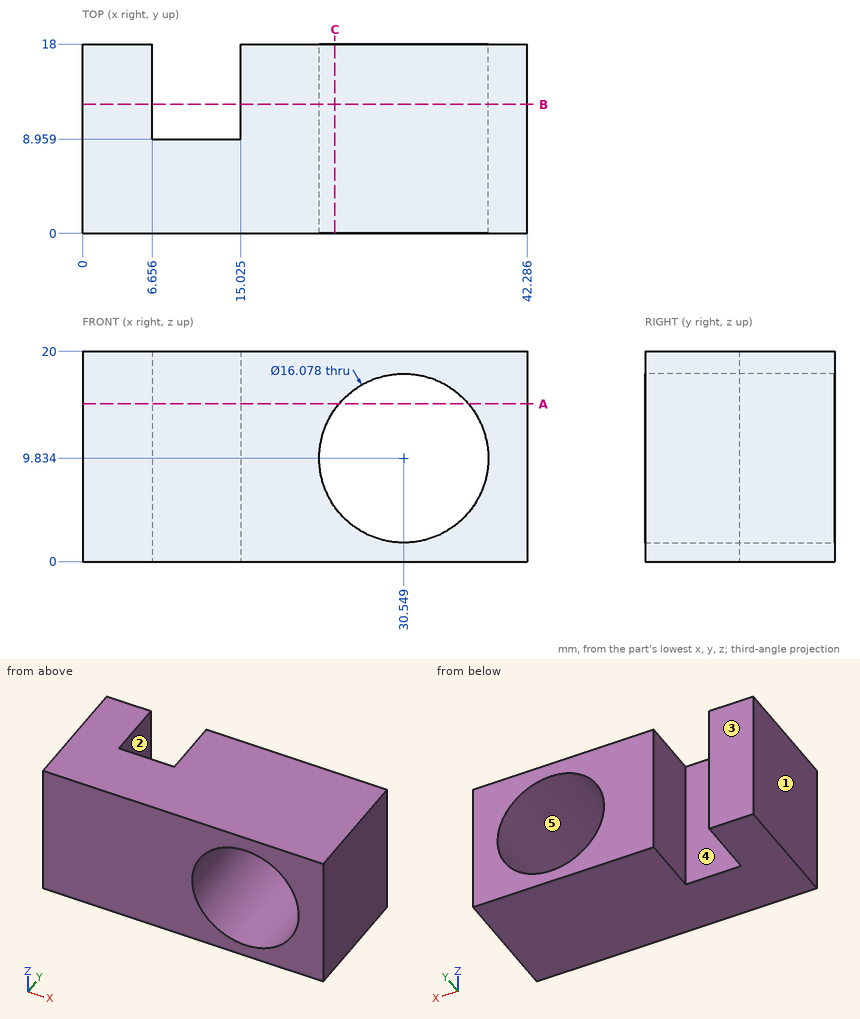
The figure shows three views and two pictorial views of one solid part (mm, origin at its lowest corner). Answer the questions. A direction names the side the tool comes from. Give positions to 0.01 mm unless a question says otherwise; leave off trailing zeros. Write each loop counter-clockwise with the first axis right and the second up, starting at its lowest first coordinate (ties: lowest second). Pieces come first, ordered by that corner, then holes. Notation, with made-up numbers: (-37, 45.5) - (12, 45.5) arc R24 ccw to (12, 63.5) - close; hole circle Ø5 at (78, 42). An arc over 180 degrees is marked (long way). Use one line per item in the form item = value.
1. Consider L1, parallel to X at y = 10, z = 9.75 (1 decimal); L2, parallel to X at y = 17, z = 18 (1 decimal); L3, parallel to X at y = 14.75, z = 7.25 (1 decimal). Determine where each line is inside the solid, lowest interval first.
Filled in:
L1 = 0 to 6.7, 15 to 22.5, 38.6 to 42.3
L2 = 0 to 6.7, 15 to 42.3
L3 = 0 to 6.7, 15 to 22.9, 38.2 to 42.3
2. Determine the mould class of the marked faces 1, 2 and 3 for opening direction X: released by +X, released by -X, zero draft, split by the parting line, or undercut.
Filled in:
face_1 = released by -X
face_2 = undercut
face_3 = zero draft
3. For the marked faces 4 and 5, determine the directions among +Z, -Z, +X, -X, +Y, -Y from which every point of the face is accessible in a straight line to the end or side of a thin tool.
Filled in:
face_4 = +Z, -Z, +Y
face_5 = +Y, -Y
4. A cutting plane is placed at B-B (y = 12.25). State how many separate pieces and enclosed holes the cut face has, and give its area (3 significant figures).
Filled in:
separate_pieces = 2
enclosed_holes = 1
area = 475 mm^2
5. This flat-tipped pin is pushed along its axis until it touches: pin 1 Ø4 at (x, z) = (9.5, 6.5) entering from +Y. Where does it stop, or does it pass through?
Filled in:
pin_1 = 8.96
6. A cutting plane is placed at A-A (z = 15). Write down the section's boundary in (x, y) (1 decimal).
Filled in:
outline = (0, 0) - (24.4, 0) - (24.4, 18) - (15, 18) - (15, 9) - (6.7, 9) - (6.7, 18) - (0, 18) - close; (36.7, 0) - (42.3, 0) - (42.3, 18) - (36.7, 18) - close
7. A cutting plane is placed at C-C (x = 24). Write down the section's boundary in (y, z) (1 decimal).
Filled in:
outline = (0, 0) - (18, 0) - (18, 5.2) - (0, 5.2) - close; (0, 14.5) - (18, 14.5) - (18, 20) - (0, 20) - close
